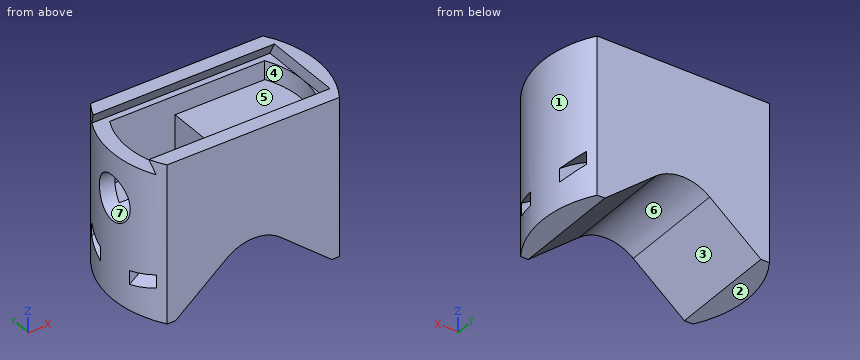
```python
from build123d import *

# Parameters (mm, degrees)
BOSS_EXTRUDE2_DEPTH      = 7
BOSS_EXTRUDE2_DEPTH_BACK = 30
CUT_EXTRUDE1_DEPTH       = 25.712971991
FILLET1_R                = 10
CUT_EXTRUDE2_START       = -17.764514
CUT_EXTRUDE2_DEPTH       = 17.764514
BOSS_EXTRUDE3_DEPTH      = 10.764514
CUT_EXTRUDE3_REACH       = 60.021
SKETCH11_R               = 5.25
SKETCH12_W               = 2.5
SKETCH12_H               = 6
CUT_EXTRUDE10_START      = -44.470309
CUT_EXTRUDE10_DEPTH      = 44.470309


with BuildPart() as part:
    # Sketch7 → Boss-Extrude2 (new, two sides)
    with BuildSketch(Plane.XY) as boss_extrude2_sk:
        with BuildLine():
            Line((-20.343909144, -12.856485995), (20.159427524, -12.856485995))
            ThreePointArc((20.159427524, -12.856485995), (23.910076333, 0), (20.159427524, 12.856485995))
            Line((20.159427524, 12.856485995), (-20.343909144, 12.856485995))
            ThreePointArc((-20.343909144, 12.856485995), (-24.06023272, 0), (-20.343909144, -12.856485995))
        make_face()
    extrude(amount=BOSS_EXTRUDE2_DEPTH)
    extrude(boss_extrude2_sk.sketch, amount=-BOSS_EXTRUDE2_DEPTH_BACK)

    # Sketch8 → Cut-Extrude1 (cut)
    with BuildSketch(Plane(origin=(0, 12.856485995, 0), x_dir=(1, 0, 0), z_dir=(0, 1, 0))):
        Polygon((-18.343909144, 30), (0, 30), (0, 15), align=None)
    cut_extrude1 = extrude(amount=-CUT_EXTRUDE1_DEPTH, mode=Mode.SUBTRACT)

    # Mirror1: Cut-Extrude1 across plane
    add(cut_extrude1.mirror(Plane(origin=(0, 0, 0), x_dir=(0, 0, 1), z_dir=(1, 0, 0))), mode=Mode.SUBTRACT)

    # Fillet1
    fillet1_edges = [part.edges().sort_by_distance(p)[0] for p in [
        (0, 0, -15),
    ]]
    fillet(fillet1_edges, radius=FILLET1_R)

    # Sketch9 → Cut-Extrude2 (cut)
    with BuildSketch(Plane.XY.offset(7).offset(CUT_EXTRUDE2_START)):
        with BuildLine():
            Line((-18.312348097, -9.356485995), (18.139112044, -9.356485995))
            ThreePointArc((18.139112044, -9.356485995), (20.410076333, 0), (18.139112044, 9.356485995))
            Line((18.139112044, 9.356485995), (-18.312348097, 9.356485995))
            ThreePointArc((-18.312348097, 9.356485995), (-20.56023272, 0), (-18.312348097, -9.356485995))
        make_face()
    extrude(amount=CUT_EXTRUDE2_DEPTH, mode=Mode.SUBTRACT)


with BuildPart() as boss_extrude3_tool:
    # Sketch10 → Boss-Extrude3 (new body)
    with BuildSketch(Plane(origin=(0, 0, -10.764513537), x_dir=(-1, 0, 0), z_dir=(0, 0, -1))):
        with BuildLine():
            Line((3.288113076, 8.856485995), (3.288113076, -8.856485995))
            Line((3.288113076, -8.856485995), (-17.831819744, -8.856485995))
            ThreePointArc((-17.831819744, -8.856485995), (-19.910076333, 0), (-17.831819744, 8.856485995))
            Line((-17.831819744, 8.856485995), (3.288113076, 8.856485995))
        make_face()
    extrude(amount=-BOSS_EXTRUDE3_DEPTH)


with BuildPart() as part_1:
    add(part.part)


with BuildPart() as part_2:
    # Boss-Extrude3: joined with boss_extrude3_tool
    add(part_1.part.fuse(boss_extrude3_tool.part, tol=0.00001))

    # Cut-Extrude3: up to this face of the body (flat: up to its plane)
    cut_extrude3_end = Plane(part_2.part.faces().sort_by_distance((-3.288113076, 0, -5.382256537))[0])
    # Sketch11 → Cut-Extrude3 (cut, up to the picked face)
    with BuildSketch(Plane.ZY.offset(24.06023272), mode=Mode.PRIVATE) as cut_extrude3_sk1:
        with Locations((-6.485, 0.212445037)):
            Circle(SKETCH11_R)
    cut_extrude3_tool1 = split(extrude(cut_extrude3_sk1.sketch, amount=-CUT_EXTRUDE3_REACH, mode=Mode.PRIVATE), bisect_by=cut_extrude3_end, keep=Keep.BOTH, mode=Mode.PRIVATE)
    add(cut_extrude3_tool1.solids().sort_by(Axis((-24.060233, 0.212445, -6.485), (1, 0, 0)))[0], mode=Mode.SUBTRACT)

    # Sketch12 → Cut-Revolve1 (revolve, cut)
    with BuildSketch(Plane(origin=(0, 0, 0), x_dir=(0, 0, -1), z_dir=(1, 0, 0))):
        with Locations((14.035, 7.856485995)):
            Rectangle(SKETCH12_W, SKETCH12_H)
        with Locations((14.035, -7.856485995)):
            Rectangle(SKETCH12_W, SKETCH12_H)
    revolve(axis=Axis((0, -85.887973373, -51.567605329), (0, 1, 0)), mode=Mode.SUBTRACT)

    # Sketch14 → Cut-Extrude10 (cut)
    with BuildSketch(Plane.ZY.offset(24.06023272).offset(CUT_EXTRUDE10_START)):
        Polygon((7, 9.356485995), (4, 10.856485995), (4, -10.856485995), (7, -9.356485995), align=None)
    extrude(amount=CUT_EXTRUDE10_DEPTH, mode=Mode.SUBTRACT)


solid = part_2.part
```
Verification items for the finished model (mm, model axes). Face numbers are marked on the shaded views. A direction names the side the tool comes from. Give positions to 0.01 mm unless a question says otherwise; leave off trailing zeros. Write each loop counter-clockwise with the first axis right and the second up, starting at its lowest first coordinate (ties: lowest second). Pieces come first, ordered by that corner, then holes. Notation, with made-up numbers: (30, 17.5) - (67, 17.5) arc R18 ccw to (67, 24.5) - close; hole circle Ø2 at (-37.5, 50.5). An arc over 180 degrees is marked (long way). Put each result on its own line as item: value.
Q1. Set-up check for the marked faces 5, 6 and 7: record each of +Z, -Z, +X, -X, +Y, -Y from which the full face is reachable in a straight line by a thin tool's end or side.
Result:
face 5: +Z
face 6: -Z, +Y, -Y
face 7: -X
Q2. Mould release check, pull along X, two halves, no side actions. Record for the marked faces 1, 2, 3 and 4: released by +X, released by -X, zero draft, split by the parting line, or undercut.
Result:
face 1: released by +X
face 2: zero draft
face 3: undercut
face 4: undercut
Q3. Section check B-B on y = -10. Record the cut outline in (x, z).
Result:
outline: (-21.89, -30) - (-18.34, -30) - (-6.33, -20.18) arc R10 cw to (6.33, -20.18) - (18.34, -30) - (21.72, -30) - (21.72, -22.5) arc R36.28 ccw to (-21.89, -22.63) - close; (-21.89, -19.55) arc R38.78 cw to (21.72, -19.44) - (21.72, 7) - (-21.89, 7) - (-21.89, 5.71) - (20.41, 5.71) - (20.41, 4) - (-21.89, 4) - close
Q4. Section check D-D on x = -7. Record the cut outline in (y, z) (3 decimals).
Result:
outline: (-12.856, -20.724) - (12.856, -20.724) - (12.856, 7) - (9.356, 7) - (10.856, 4) - (9.356, 4) - (9.356, -10.765) - (3.254, -10.765) arc R5.25 cw to (-2.829, -10.765) - (-9.356, -10.765) - (-9.356, 4) - (-10.856, 4) - (-9.356, 7) - (-12.856, 7) - close; hole (-10.856, -15.967) - (-4.856, -15.967) - (-4.856, -13.422) - (-10.856, -13.422) - close; hole (4.856, -15.967) - (10.856, -15.967) - (10.856, -13.422) - (4.856, -13.422) - close
Q5. Section check A-A on z = 3. Record the cut outline in (x, y), and give its area (3 significant figures).
Result:
outline: (-20.34, -12.86) - (20.16, -12.86) arc R23.91 ccw to (20.16, 12.86) - (-20.34, 12.86) arc R24.1 ccw to start; hole (-18.31, -9.36) - (18.14, -9.36) arc R20.41 ccw to (18.14, 9.36) - (-18.31, 9.36) arc R20.6 ccw to start
area: 432 mm2
Q6. Section check C-C on z = -4. Record the cut outline in (x, y).
Result:
outline: (-23.65, -4.41) arc R24.1 ccw to (-20.34, -12.86) - (20.16, -12.86) arc R23.91 ccw to (20.16, 12.86) - (-20.34, 12.86) arc R24.1 ccw to (-23.57, 4.84) - (-19.98, 4.84) arc R20.6 cw to (-18.31, 9.36) - (18.14, 9.36) arc R20.41 cw to (18.14, -9.36) - (-18.31, -9.36) arc R20.6 cw to (-20.08, -4.41) - close; (-3.29, -8.86) - (17.83, -8.86) arc R19.91 ccw to (17.83, 8.86) - (-3.29, 8.86) - close
Q7. Scan lines: probe 1 along Y at (x, z) = (-7.5, -14); probe 2 along Y at (x, z) = (1, -4); probe 3 along Y at (x, z) = (17, 3). Record each from-to range of solid material in increasing order. Write a range as from..to.
Result:
probe 1: -12.86..-10.86, -4.86..4.86, 10.86..12.86
probe 2: -12.86..-9.36, -8.86..8.86, 9.36..12.86
probe 3: -12.86..-9.36, 9.36..12.86
Q8. Depth check by flat-ended pin: P1, Ø9, axis at x = 5, y = 2.5, coming from the +Z side; P2, Ø1.5, axis at y = 0, z = -1.5, coming from the -X side; P3, Ø4, axis at x = 13.5, y = 1.5, coming from the -Z side; P4, Ø1, axis at y = 3, z = -10, coming from the +X side. Enter the tip coordinate at first touch or a pass-through.
Result:
P1: z = 0
P2: x = -24.06
P3: z = -27.67
P4: x = 23.78
